```python
from build123d import *

# Parameters (mm, degrees)
SKETCH_1_R          = 1.1
SKETCH_1_W          = 74
SKETCH_1_H          = 57
EXTRUDE_1_DEPTH     = 28
SKETCH_2_W          = 40
SKETCH_2_H          = 14
CUT_EXTRUDE_1_DEPTH = 28
CUT_EXTRUDE_2_DEPTH = 90.388198326
CUT_EXTRUDE_5_DEPTH = 59.542719445
EXTRUDE_2_DEPTH     = 28
FILLET_1_R          = 1
FILLET_2_R          = 1
FILLET_3_R          = 10
CUT_EXTRUDE_6_REACH = 82.006
CUT_EXTRUDE_7_REACH = 91.388


with BuildPart() as part:
    # 草图1 → 凸台-拉伸1 (new body)
    with BuildSketch(Plane(origin=(0, 0, 0), x_dir=(1, 0, 0), z_dir=(0, 1, 0))):
        Polygon((-39, -30.5), (39, -30.5), (39, 30.5), (39, 33.5), (-39, 33.5), (-39, 30.5), align=None)
        with Locations(Location((24, 31, 0), (0, 0, 270))):
            Circle(SKETCH_1_R, mode=Mode.SUBTRACT)
        with Locations(Location((-24, 31, 0), (0, 0, 270))):
            Circle(SKETCH_1_R, mode=Mode.SUBTRACT)
        Rectangle(SKETCH_1_W, SKETCH_1_H, mode=Mode.SUBTRACT)
    extrude(amount=EXTRUDE_1_DEPTH)

    # 草图2 → 切除-拉伸1 (cut)
    with BuildSketch(Plane(origin=(0, 28, 0), x_dir=(1, 0, 0), z_dir=(0, 1, 0))):
        with Locations((0, -30.5)):
            Rectangle(SKETCH_2_W, SKETCH_2_H)
    extrude(amount=-CUT_EXTRUDE_1_DEPTH, mode=Mode.SUBTRACT)

    # 草图3 → 切除-拉伸2 (cut, through all)
    with BuildSketch(Plane(origin=(39, 0, 0), x_dir=(0, 0, -1), z_dir=(1, 0, 0))):
        Polygon((-30.5, 28), (-14.5, 28), (-30.5, 16), align=None)
    extrude(amount=-CUT_EXTRUDE_2_DEPTH, mode=Mode.SUBTRACT)

    # 草图4 → 切除-拉伸5 (cut, through all)
    with BuildSketch(Plane(origin=(0, 28, 0), x_dir=(1, 0, 0), z_dir=(0, 1, 0))):
        Polygon((-37, -14.5), (-37, -36.587874711), (-17, -36.587874711), (-17, -15.951475091), align=None)
    extrude(amount=-CUT_EXTRUDE_5_DEPTH, mode=Mode.SUBTRACT)

    # 草图5 → 凸台-拉伸2 (add)
    with BuildSketch(Plane.ZY.offset(-20)):
        Polygon((30.5, 0), (30.5, 16), (28.5, 17.5), (28.5, 0), align=None)
    extrude(amount=EXTRUDE_2_DEPTH)

    # 圆角1
    fillet_1_edges = [part.edges().sort_by_distance(p)[0] for p in [
        (-39, 14, -33.5),
        (39, 14, -33.5),
        (39, 8, 30.5),
        (-39, 8, 30.5),
    ]]
    fillet(fillet_1_edges, radius=FILLET_1_R)

    # 圆角2
    fillet_2_edges = [part.edges().sort_by_distance(p)[0] for p in [
        (37, 14, -28.5),
        (-37, 14, -28.5),
        (37, 8.75, 28.5),
    ]]
    fillet(fillet_2_edges, radius=FILLET_2_R)

    # 圆角3
    fillet_3_edges = [part.edges().sort_by_distance(p)[0] for p in [
        (-38, 28, 14.5),
        (38, 28, 14.5),
    ]]
    fillet(fillet_3_edges, radius=FILLET_3_R)

    # 草图8 → 切除-拉伸6 (cut, up to next)
    with BuildSketch(Plane(origin=(0, 0, -33.5), x_dir=(-1, 0, 0), z_dir=(0, 0, -1)), mode=Mode.PRIVATE) as cut_extrude_6_sk1:
        Polygon((29, 28), (-29, 28), (-25, 18), (25, 18), align=None)
    cut_extrude_6_tool1 = extrude(cut_extrude_6_sk1.sketch, amount=-CUT_EXTRUDE_6_REACH, mode=Mode.PRIVATE) & part.part
    add(cut_extrude_6_tool1.solids().sort_by_distance((0, 23.123457, -33.5))[0], mode=Mode.SUBTRACT)

    # 草图9 → 切除-拉伸7 (cut, up to next)
    with BuildSketch(Plane(origin=(39, 0, 0), x_dir=(0, 0, -1), z_dir=(1, 0, 0)), mode=Mode.PRIVATE) as cut_extrude_7_sk1:
        with BuildLine():
            Line((-7.308033396, 20.191966604), (-17.5, 10))
            Line((-17.5, 10), (-5.5, 10))
            Line((-5.5, 10), (-3.5, 12))
            Line((-3.5, 12), (-12.671572875, 12))
            Line((-12.671572875, 12), (-6.064971157, 18.606601718))
            Line((-6.064971157, 18.606601718), (1.606601718, 18.606601718))
            Line((1.606601718, 18.606601718), (3.606601718, 20.606601718))
            Line((3.606601718, 20.606601718), (-6.307015681, 20.606601718))
            ThreePointArc((-6.307015681, 20.606601718), (-6.848762564, 20.498841563), (-7.308033396, 20.191966604))
        make_face()
    cut_extrude_7_tool1 = extrude(cut_extrude_7_sk1.sketch, amount=-CUT_EXTRUDE_7_REACH, mode=Mode.PRIVATE) & part.part
    # 草图9 → 切除-拉伸7 (cut, up to next)
    with BuildSketch(Plane(origin=(39, 0, 0), x_dir=(0, 0, -1), z_dir=(1, 0, 0)), mode=Mode.PRIVATE) as cut_extrude_7_sk2:
        with BuildLine():
            Line((6.606601718, 19.851812513), (6.606601718, 10))
            Line((6.606601718, 10), (9.435028843, 10))
            Line((9.435028843, 10), (20.04163056, 20.606601718))
            Line((20.04163056, 20.606601718), (17.799586037, 20.606601718))
            ThreePointArc((17.799586037, 20.606601718), (17.257839153, 20.498841563), (16.798568322, 20.191966604))
            Line((16.798568322, 20.191966604), (8.606601718, 12))
            Line((8.606601718, 12), (8.606601718, 20.606601718))
            Line((8.606601718, 20.606601718), (7.361390923, 20.606601718))
            ThreePointArc((7.361390923, 20.606601718), (6.827674357, 20.385529078), (6.606601718, 19.851812513))
        make_face()
    cut_extrude_7_tool2 = extrude(cut_extrude_7_sk2.sketch, amount=-CUT_EXTRUDE_7_REACH, mode=Mode.PRIVATE) & part.part
    # 草图9 → 切除-拉伸7 (cut, up to next)
    with BuildSketch(Plane(origin=(39, 0, 0), x_dir=(0, 0, -1), z_dir=(1, 0, 0)), mode=Mode.PRIVATE) as cut_extrude_7_sk3:
        Polygon((-6.921215742, 16.053300859), (-8.421215742, 14.553300859), (-3.421215742, 14.553300859), (-1.921215742, 16.053300859), align=None)
    cut_extrude_7_tool3 = extrude(cut_extrude_7_sk3.sketch, amount=-CUT_EXTRUDE_7_REACH, mode=Mode.PRIVATE) & part.part
    add(cut_extrude_7_tool1.solids().sort_by_distance((39, 14.928952, 12.236985))[0], mode=Mode.SUBTRACT)
    add(cut_extrude_7_tool2.solids().sort_by_distance((39, 14.925906, -6.777774))[0], mode=Mode.SUBTRACT)
    add(cut_extrude_7_tool3.solids().sort_by_distance((39, 15.303301, 5.171216))[0], mode=Mode.SUBTRACT)


solid = part.part
```
Check sheet for the modelled part. Datum: model origin and axes. Units: mm. A direction names the side the tool comes from. Coordinates: 2 decimals unless noted, no trailing zeros. Order: outer loops, then holes, each group sorted by start corner. A loop starts at its lowest first (then second) coordinate and runs counter-clockwise, first axis right, second up. Notation, with made-up numbers: M -31,83.5 L 27,83.5 A22 ccw 27,102.5 Z; hole C 3.5,82 d8. An arc over 180 degrees is marked long. One line per question, with ' | ' between items. Start each with the question number.
Item 1: Gauge pin test, flat ends, axial feed: P1, Ø0.6, axis at x = 38.5, y = 12.5, coming from the -Z side; P2, Ø1.5, axis at x = -1, z = -26, coming from the +Y side; P3, Ø3, axis at x = 24, z = -31, coming from the +Y side. Record the tip position at first contact, or that the pin passes through.
Item 2: Mould release check, pull along Z, two halves, no side actions. Record for faces 1 (the cylindrical face through (-38.01, 27.5, 14.29)), 2 (the flat face through (38, 20.607, -19)), 3 (the flat face through (39, 14, -1)): pulls with the +Z half, pulls with the -Z half, needs draft (parallel to the pull), parting line crosses it, or undercut.
Item 3: Sectioned sample at D-D on z = 25. Record the cut outline in (x, y) (3 decimals), and give its area (3 significant figures).
Item 4: Sectioned sample at A-A on y = 3.25. Record the cut outline in (x, z), and give its area (3 significant figures).
Item 5: Material ranges on line 1 (X direction, y = 12.5, z = -31); line 2 (Z direction, x = 24, y = 5.5); line 3 (X direction, y = 14.25, z = 25), recorded low to high.
Item 6: Sectioned sample at B-B on x = -24. Record the cut outline in (y, z).
Item 7: Access from +Z, -Z, +X, -X, +Y, -Y to the whole of each face (thin tool, end or side, straight path). Record for faces 4 (the flat face through (38, 10, 12)), 5 (the flat face through (0, 18, -31)), 6 (the flat face through (-37, 14, 1)), 7 (the flat face through (37.3, 28, -17.9)), 8 (the flat face through (37, 14, 0)).
Item 8: Sectioned sample at C-C on x = 24. Record the cut outline in (y, z), and give its area (3 significant figures).
Answer below:
1) P1: stops at z = -33.48 | P2: passes through | P3: stops at y = 19.25
2) face 1: pulls with the +Z half | face 2: undercut | face 3: needs draft
3) outline: M -39,0 L -37,0 L -37,20.125 L -39,20.125 Z; M 37,0 L 39,0 L 39,20.125 L 37,20.125 Z | area: 80.5 mm^2
4) outline: M -39,-32.5 A1 ccw -38,-33.5 L 38,-33.5 A1 ccw 39,-32.5 L 39,29.5 A1 ccw 38,30.5 L -8,30.5 L -8,28.5 L 36,28.5 A1 cw 37,27.5 L 37,-27.5 A1 cw 36,-28.5 L -36,-28.5 A1 cw -37,-27.5 L -37,30.5 L -38,30.5 A1 ccw -39,29.5 Z; hole C -24,-31 d2.2; hole C 24,-31 d2.2 | area: 708 mm^2
5) line 1: x = -39 to -25.1, -22.9 to 22.9, 25.1 to 39 | line 2: z = -33.5 to -32.1, -29.9 to -28.5, 28.5 to 30.5 | line 3: x = -39 to -37, 37 to 39
6) outline: M 0,-33.5 L 18,-33.5 L 18,-32.1 L 0,-32.1 Z; M 0,-29.9 L 18,-29.9 L 18,-28.5 L 0,-28.5 Z
7) face 4: +X | face 5: +Z, -Z, +Y | face 6: +Z, +Y, -Y | face 7: +Z, -Z, +X, -X, +Y | face 8: +Y, -Y
8) outline: M 0,-33.5 L 18,-33.5 L 18,-32.1 L 0,-32.1 Z; M 0,-29.9 L 18,-29.9 L 18,-28.5 L 0,-28.5 Z; M 0,28.5 L 17.5,28.5 L 16,30.5 L 0,30.5 Z | area: 83.9 mm^2
